Model file for the job. Use its own axes, mm. Face numbers are marked on the shaded views. Give positions to 0.01 mm unless a question says otherwise; leave off trailing zeros. Write each loop counter-clockwise with the first axis right and the second up, starting at its lowest first coordinate (ties: lowest second). Pieces come first, ordered by that corner, then holes. Notation, with made-up numbers: M 86.25,-22 L 95.25,-22 A28 ccw 95.25,4 Z; hole C 73.5,56.5 d6. An arc over 180 degrees is marked long. Answer as a JSON object with one key per item and string values. Group by question number.
Autodesk Inventor part; units mm, degrees
ref_plane "YZ Plane" through (0, 0, 0) normal (1, 0, 0) x (0, 1, 0)
ref_plane "XZ Plane" through (0, 0, 0) normal (0, 1, 0) x (-1, 0, 0)
ref_plane "XY Plane" through (0, 0, 0) normal (0, 0, 1) x (1, 0, 0)
sketch "Boceto1" plane through (0, 0, 0) normal (0, 0, 1) x (1, 0, 0)
  circle A0 centre (0, 0) radius 4
  line L0 (-37.8416, 0) -> (37.8416, 0) construction
  line L1 (0, 25.1226) -> (0, -25.1226) construction
  line L2 (-4.25, 5) -> (4.25, 5)
  line L3 (-4.25, -5) -> (4.25, -5)
  line L4 (-4.25, 5) -> (-6, 0)
  line L5 (-4.25, -5) -> (-6, 0)
  line L6 (4.25, 5) -> (6, 0)
  line L7 (4.25, -5) -> (6, 0)
  point P0 (0, 5)
  point P1 (0, -5)
  dimension "d0" = 8
  dimension "d1" = 8.5
  dimension "d2" = 8.5
  dimension "d3" = 5
  dimension "d4" = 5
  dimension "d5" = 6
  dimension "d6" = 6
extrude "Extrusión1" add sketch "Boceto1" against normal blind 6
thread "Rosca1"
chamfer "Chaflán1" distance 0.5 angle 45 1 edges at (-4, 0, 0)
chamfer "Chaflán2" distance 0.5 angle 45 1 edges at (-4, 0, -6)
equation "\"d2\" = d1"
equation "\"d4\" = d3"
properties part number "2-HUDSON-8-35-TDR HAND PUMP M8x5 PIPE NU"
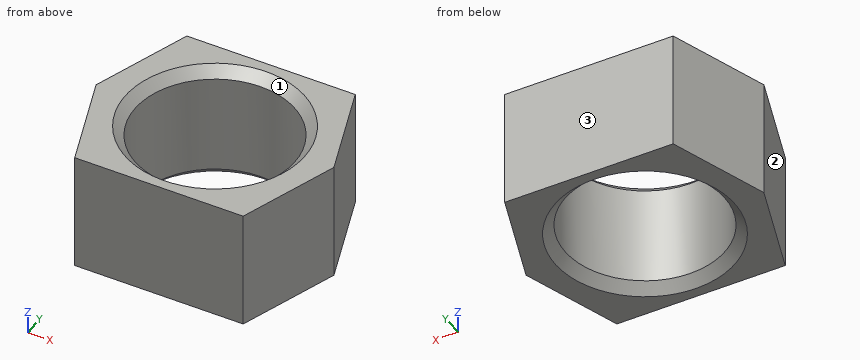
Q1. Slice it at A-A, the plane z = -3. Write the cut outline in (x, y), then the cut area to 3 significant figures.
Q2. Wall check: L1, parallel to Y at x = 0, z = -1.55; L2, parallel to X at y = -2.75, z = -0.6; L3, parallel to X at y = 2.5, z = -3 (1 decimal). Give the ranges that are in metal, low to high.
Q3. Slice it at B-B, the plane x = 0. Write the cut outline in (y, z).
Q4. Two-plate mould, pull along X, no slides. Class the marked faces 1, 2 and 3: +X half, -X half, draft (parallel to the pull), parting line (faces both ways), or undercut.
Q5. Drop flat-ended pins along their axis: P1, Ø1, axis at y = -3.5, z = -1, coming from the -X side; P2, Ø4, axis at x = -2.5, y = -3.5, coming from the +Z side. Give the stop position or say it passes through.
Solved:
{
 "1": {"outline": "M -6,0 L -4.25,-5 L 4.25,-5 L 6,0 L 4.25,5 L -4.25,5 Z; hole C 0,0 d8", "area": "52.2 mm²"},
 "2": {"L1": "y = -5 to -4, 4 to 5", "L2": "x = -5.04 to -2.9, 2.9 to 5.04", "L3": "x = -5.1 to -3.1, 3.1 to 5.1"},
 "3": {"outline": "M -5,-6 L -4.5,-6 L -4,-5.5 L -4,-0.5 L -4.5,0 L -5,0 Z; M 4,-5.5 L 4.5,-6 L 5,-6 L 5,0 L 4.5,0 L 4,-0.5 Z"},
 "4": {"face 1": "undercut", "face 2": "-X half", "face 3": "draft"},
 "5": {"P1": "stops at x = -4.95", "P2": "stops at z = 0"}
}
